from build123d import *

# Parameters (mm, degrees)
F0_R     = 8.9
F1_DEPTH = 2
F0_R_2   = 11
F2_DEPTH = 10.5
F3_R     = 2


with BuildPart() as f1:
    # F0 (on Top) → F1 (new body)
    with BuildSketch(Plane.XY):
        Circle(F0_R)
    extrude(amount=F1_DEPTH)

    # F0 (on Top) → F2 (join)
    with BuildSketch(Plane.XY):
        Circle(F0_R_2)
        Circle(F0_R, mode=Mode.SUBTRACT)
    extrude(amount=F2_DEPTH)

    # F3
    f3_edges = [f1.edges().sort_by_distance(p)[0] for p in [
        (-11, 0, 0),
    ]]
    fillet(f3_edges, radius=F3_R)


solid = f1.part
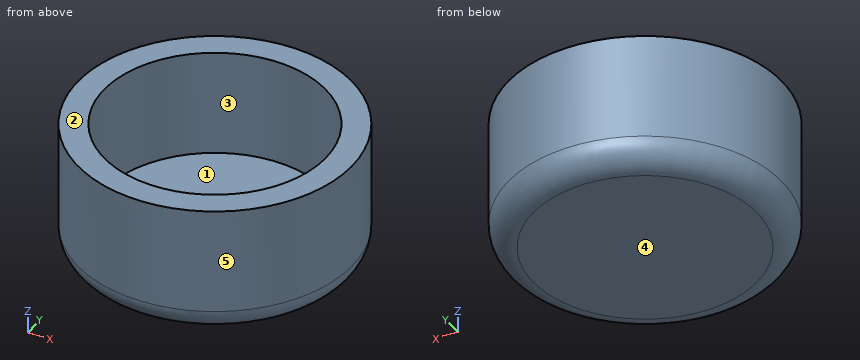
Can you work these out from the model? Positions are in its coordinate system, mm. Face numbers are marked on the shaded views. A direction names the side the tool comes from. Give positions to 0.01 mm unless a question says otherwise; leave off trailing zeros. Order: outer loops, then holes, each group sorted by start corner. A loop starts at its lowest first (then second) coordinate and runs counter-clockwise, first axis right, second up. Notation, with made-up numbers: M 79,83 L 92,83 A21 ccw 92,102 Z; hole C 77,72.5 d8. An arc over 180 degrees is marked long. One line per item, written item: value.
Item 1: Please list where these lines run through material, in increasing order: line 1 (Y direction, x = 0, z = 4.5); line 2 (Z direction, x = -4.5, y = -1.75); line 3 (Z direction, x = 1.75, y = -9).
Verdict:
line 1: -11 to -8.9, 8.9 to 11
line 2: 0 to 2
line 3: 0.01 to 10.5
Item 2: If we section it at B-B on z = 6.5: Write out the boundary of the cut face in (x, y), and give its area (3 significant figures).
Verdict:
outline: C 0,0 d22; hole C 0,0 d17.8
area: 131 mm2
Item 3: If we section it at A-A on y = 0: Write out the boundary of the cut face in (x, z), and give its area (3 significant figures).
Verdict:
outline: M -11,2 A2 ccw -9,0 L 9,0 A2 ccw 11,2 L 11,10.5 L 8.9,10.5 L 8.9,2 L -8.9,2 L -8.9,10.5 L -11,10.5 Z
area: 78.0 mm2
Item 4: For pin 1 (4 mm diameter, centred on y = -3.5, z = 9.5, fed in from +X); pin 2 (5 mm diameter, centred on x = -5, z = 8.5, fed in from +Y); pin 3 (4 mm diameter, centred on x = 8, z = 4.5, fed in from +Y); pin 4 (9 mm diameter, centred on x = 2.5, y = -4, fed in from +Z), each with a flat end and sliding along its axis, tell me the tip position at first contact or that it passes through.
Verdict:
pin 1: x = 10.9
pin 2: y = 10.71
pin 3: y = 9.22
pin 4: z = 10.5
Item 5: If we mould it in two halves opening along X, with no side actions, what happens to the marked faces 3, 4 and 5? For each: pulls with the +X half, pulls with the -X half, needs draft (parallel to the pull), parting line crosses it, or undercut.
Verdict:
face 3: undercut
face 4: needs draft
face 5: parting line crosses it
Item 6: For the marked faces 1 and 2, which set-ups out of +Z, -Z, +X, -X, +Y, -Y let a thin tool reach every point of the face, with its end or its side?
Verdict:
face 1: +Z
face 2: +Z, +X, -X, +Y, -Y
